The listing builds one solid part. Answer for the finished solid, in the listing's coordinates (mm). A direction names the side the tool comes from. Give positions to 0.01 mm unless a question says otherwise; leave off trailing zeros. Order: outer loops, then holes, each group sorted by start corner. A loop starts at its lowest first (then second) coordinate and runs counter-clockwise, first axis right, second up. Notation, with made-up numbers: (59, 1.5) -> (68, 1.5) arc R18 cw to (68, 13.5) -> close; hole circle Ø1 at (-25.75, 6). An arc over 180 degrees is marked (long way). Write item = value, one per line. Start each with the question number.
```python
from build123d import *

# Parameters (mm, degrees)
SKETCH1_R           = 3
SKETCH1_R_2         = 1.25
BOSS_EXTRUDE1_DEPTH = 5
BOSS_EXTRUDE2_START = -1.5
SKETCH2_R           = 3
SKETCH2_R_2         = 1.5
BOSS_EXTRUDE2_DEPTH = 1.5


with BuildPart() as part:
    # Sketch1 → Boss-Extrude1 (new body)
    with BuildSketch(Plane.XY):
        with BuildLine():
            Line((-6.599663291, -2.333333333), (-1.885618083, -15.666666667))
            ThreePointArc((-1.885618083, -15.666666667), (0, -17), (1.885618083, -15.666666667))
            Line((1.885618083, -15.666666667), (6.599663291, -2.333333333))
            ThreePointArc((6.599663291, -2.333333333), (7, 0), (6.599663291, 2.333333333))
            Line((6.599663291, 2.333333333), (1.885618083, 15.666666667))
            ThreePointArc((1.885618083, 15.666666667), (0, 17), (-1.885618083, 15.666666667))
            Line((-1.885618083, 15.666666667), (-6.599663291, 2.333333333))
            ThreePointArc((-6.599663291, 2.333333333), (-7, 0), (-6.599663291, -2.333333333))
        make_face()
        Circle(SKETCH1_R, mode=Mode.SUBTRACT)
        with Locations((0, 15)):
            Circle(SKETCH1_R_2, mode=Mode.SUBTRACT)
        with Locations((0, -15)):
            Circle(SKETCH1_R_2, mode=Mode.SUBTRACT)
    extrude(amount=BOSS_EXTRUDE1_DEPTH)

    # Sketch2 → Boss-Extrude2 (add)
    with BuildSketch(Plane.XY.offset(5).offset(BOSS_EXTRUDE2_START)):
        Circle(SKETCH2_R)
        Circle(SKETCH2_R_2, mode=Mode.SUBTRACT)
    extrude(amount=BOSS_EXTRUDE2_DEPTH)


solid = part.part
```
Item 1: The mould has two halves that part along X. Classify faces 3 (the cylindrical face through (0, -17, 2)), 4 (the cylindrical face through (0.672, 16.054, 2.465)), 5 (the flat face through (-4.276, -8.907, 2.465)): +X half, -X half, draft (parallel to the pull), parting line (faces both ways), or undercut.
Item 2: A cutting plane is placed at B-B, the plane x = 0. Write down the section's boundary in (y, z), plus the area to 4 significant figures.
Item 3: A cutting plane is placed at C-C, the plane y = -1. Write down the section's boundary in (x, z), plus the area to 3 significant figures.
Item 4: Flat-ended cylindrical pins translate along their axes: pin 1 (3 mm diameter, centred on x = 1.5, y = -6, fed in from -Z); pin 2 (1 mm diameter, centred on x = 1, z = 4.5, fed in from -Y). Find the tip coordinate at first contact, or state that the pin passes through.
Item 5: Consider L1, parallel to Y at x = 0, z = 4.5; L2, parallel to Z at x = 2, y = -1; L3, parallel to X at y = 8, z = 3.95. Determine where each line is inside the solid, lowest interval first. Write a range as from..to.
Item 6: A cutting plane is placed at A-A, the plane z = 4.65. Write down the section's boundary in (x, y), plus the area to 3 significant figures.
Item 7: A cutting plane is placed at D-D, the plane z = 1.8. Write down the section's boundary in (x, y), plus the area to 3 significant figures.
Item 8: Which of the six approach directions +Z, -Z, +X, -X, +Y, -Y give full straight-line access (tool end or side, diameter ignored) to faces 1 (the flat face through (-2, 0, 5)), 2 (the cylindrical face through (-3, 0, 2))?
Check values:
q1.face_3 = parting line
q1.face_4 = undercut
q1.face_5 = -X half
q2.outline = (-17, 0) -> (-16.25, 0) -> (-16.25, 5) -> (-17, 5) -> close; (-13.75, 0) -> (-3, 0) -> (-3, 3.5) -> (-1.5, 3.5) -> (-1.5, 5) -> (-13.75, 5) -> close; (1.5, 3.5) -> (3, 3.5) -> (3, 0) -> (13.75, 0) -> (13.75, 5) -> (1.5, 5) -> close; (16.25, 0) -> (17, 0) -> (17, 5) -> (16.25, 5) -> close
q2.area = 119.5 mm^2
q3.outline = (-6.93, 0) -> (-2.83, 0) -> (-2.83, 3.5) -> (-1.12, 3.5) -> (-1.12, 5) -> (-6.93, 5) -> close; (1.12, 3.5) -> (2.83, 3.5) -> (2.83, 0) -> (6.93, 0) -> (6.93, 5) -> (1.12, 5) -> close
q3.area = 46.1 mm^2
q4.pin_1 = 0
q4.pin_2 = -16.94
q5.L1 = -17..-16.25, -13.75..-1.5, 1.5..13.75, 16.25..17
q5.L2 = 3.5..5
q5.L3 = -4.6..4.6
q6.outline = (-6.6, -2.33) -> (-1.89, -15.67) arc R2 ccw to (1.89, -15.67) -> (6.6, -2.33) arc R7 ccw to (6.6, 2.33) -> (1.89, 15.67) arc R2 ccw to (-1.89, 15.67) -> (-6.6, 2.33) arc R7 ccw to start; hole circle Ø3 at (0, 0); hole circle Ø2.5 at (0, -15); hole circle Ø2.5 at (0, 15)
q6.area = 281 mm^2
q7.outline = (-6.6, -2.33) -> (-1.89, -15.67) arc R2 ccw to (1.89, -15.67) -> (6.6, -2.33) arc R7 ccw to (6.6, 2.33) -> (1.89, 15.67) arc R2 ccw to (-1.89, 15.67) -> (-6.6, 2.33) arc R7 ccw to start; hole circle Ø6 at (0, 0); hole circle Ø2.5 at (0, -15); hole circle Ø2.5 at (0, 15)
q7.area = 260 mm^2
q8.face_1 = +Z, +X, -X, +Y, -Y
q8.face_2 = -Z
